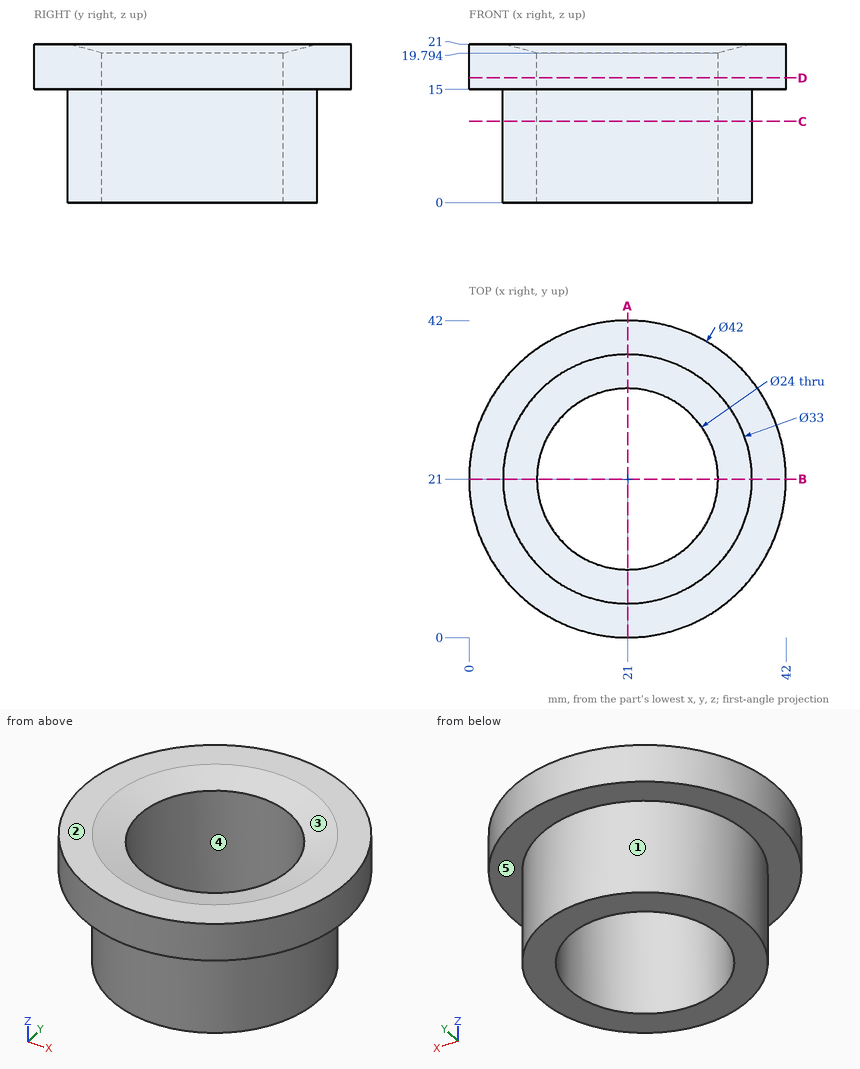
Job drawing, mm, ordinate dimensions from the low corner. One solid piece. A direction names the side the tool comes from. Give positions to 0.01 mm unless a question says otherwise; leave off trailing zeros. Loops run counter-clockwise (first coordinate to the right, second up) from the corner with the lowest first, then second, coordinate; pieces in that order, holes last. Notation, with made-up numbers: M 87,-36.75 L 95,-36.75 A10 cw 95,-17.75 Z; hole C -1.75,-23 d4. An arc over 180 degrees is marked long. Answer in a Markdown table with one row per item. Add a question column.
Item 1: Probe probe 1 along Y at (x, z) = (21, 12.25); probe 2 along Y at (x, z) = (21, 15.25); probe 3 along Z at (x, y) = (36, 30). List the from-to ranges inside material, lowest first.
Item 2: Drop flat-ended pins along their axis: P1, Ø10, axis at x = 24.5, y = 34, coming from the -Z side; P2, Ø5, axis at y = 14.5, z = 17, coming from the +X side; P3, Ø8, axis at x = 6.5, z = 9.5, coming from the -Y side; P4, Ø6, axis at x = 8, z = 5, coming from the +Y side (1 decimal). Give the stop position or say it passes through.
Item 3: Band-saw the part on C-C on z = 10.75. Give the cut face in (x, y), then the cut area to 3 significant figures.
Item 4: Tool access for the marked faces 4 and 5: list every direction of +Z, -Z, +X, -X, +Y, -Y with a clear straight run to the whole face (end or side of a thin tool).
Item 5: Band-saw the part on A-A on x = 21. Give the cut face in (y, z).
Item 6: Mould opens along Y. For the marked faces 1, 2 and 3 say: +Y half, -Y half, draft (parallel to the pull), parting line (faces both ways), or undercut.
Item 7: Band-saw the part on D-D on z = 16.5. Give the cut face in (x, y).
Reply:
| question | item | result |
|---|---|---|
| 1 | probe 1 | y = 4.5 to 9, 33 to 37.5 |
| 1 | probe 2 | y = 0 to 9, 33 to 42 |
| 1 | probe 3 | z = 15 to 21 |
| 2 | P1 | stops at z = 0 |
| 2 | P2 | stops at x = 41.62 |
| 2 | P3 | stops at y = 8.27 |
| 2 | P4 | stops at y = 34.1 |
| 3 | outline | C 21,21 d33; hole C 21,21 d24 |
| 3 | area | 403 mm^2 |
| 4 | face 4 | +Z, -Z |
| 4 | face 5 | -Z |
| 5 | outline | M 0,15 L 4.5,15 L 4.5,0 L 9,0 L 9,19.79 L 4.5,21 L 0,21 Z; M 33,0 L 37.5,0 L 37.5,15 L 42,15 L 42,21 L 37.5,21 L 33,19.79 Z |
| 6 | face 1 | parting line |
| 6 | face 2 | draft |
| 6 | face 3 | undercut |
| 7 | outline | C 21,21 d42; hole C 21,21 d24 |
